Build history of the part. All positions in model axes, mm. A direction names the side the tool comes from. Round coordinates to 2 decimals unless told otherwise and drop trailing zeros. Write each loop counter-clockwise with the first axis right and the second up, starting at its lowest first coordinate (ties: lowest second). Pieces come first, ordered by that corner, then holes. Notation, with made-up numbers: (-35.5, 0.5) - (-10.5, 0.5) arc R18 cw to (-10.5, 17.5) - close; hole circle Ø2 at (55.5, 20). An arc over 180 degrees is marked (long way). Write each question's results on one line, items separated by ' | '.
from build123d import *

# Parameters (mm, degrees)
F0_W      = 90.9466184676
F0_H      = 74.8294964433
F2_DEPTH  = 5.08
F3_DEPTH  = 50.8
F5_DEPTH  = 76.2
F6_DEPTH  = 25.4
F8_DEPTH  = 101.6
F9_R      = 2.2127457179
F9_R_2    = 2.6181554233
F9_R_3    = 2.4324763665
F9_R_4    = 2.5640554726
F10_DEPTH = 25.4


with BuildPart() as f2:
    # F0 (on Front) → F2 (new body)
    with BuildSketch(Plane.XZ):
        with Locations((8.6341705173, 1.7268359661)):
            Rectangle(F0_W, F0_H)
    extrude(amount=F2_DEPTH)

    # F1 (on face) → F3 (join)
    with BuildSketch(Plane.XZ):
        Polygon((-27.9171578586, 32.2342440486), (-36.8391387165, 32.2342440486), (-36.8391387165, 2.734344452), (-36.5513302386, -26.7659369856), (-26.765935123, -26.7659369856), (-26.765935123, -34.8244979978), (43.1708656251, -34.8244979978), (43.1708656251, -26.4781285077), (54.1074797511, -26.4781285077), (54.1074797511, 31.0830231756), (42.5952523947, 31.0830231756), (42.5952523947, 39.1415841877), (-27.9171578586, 39.1415841877), align=None)
    extrude(amount=-F3_DEPTH)

    # F4 (on face) → F5 (cut)
    with BuildSketch(Plane.XY.offset(39.1415841877)):
        Polygon((-27.9171578586, 50.8), (-27.9171578586, 30.387243256), (12.6576088369, 14.234690927), (42.5952523947, 50.8), align=None)
    extrude(amount=-F5_DEPTH, mode=Mode.SUBTRACT)

    # F6 (cut): a face of the model
    f6_faces = [f2.faces().sort_by_distance(p)[0] for p in [
        (-32.3426594813, 50.8, 2.8940476275),
    ]]
    extrude(f6_faces, amount=-F6_DEPTH, mode=Mode.SUBTRACT)

    # F7 (on face) → F8 (cut)
    with BuildSketch(Plane(origin=(0, 0, -34.8244979978), x_dir=(1, 0, 0), z_dir=(0, 0, -1))):
        Polygon((-24.7789256071, -18.5888221988), (-22.6721912622, -24.9785389751), (9.4293939445, -12.1991054226), (6.9454660549, -5.9595469581), align=None)
    extrude(amount=-F8_DEPTH, mode=Mode.SUBTRACT)

    # F9 (on face) → F10 (cut)
    with BuildSketch(Plane(origin=(0, 0, 0), x_dir=(-1, 0, 0), z_dir=(0, 1, 0))):
        with Locations((32.3781482875, 36.15520522)):
            Circle(F9_R)
        with Locations((32.3781482875, -30.7667031884)):
            Circle(F9_R_2)
        with Locations((-49.00373891, -31.279515475)):
            Circle(F9_R_3)
        with Locations((-49.5165549219, 36.15520522)):
            Circle(F9_R_4)
    extrude(amount=-F10_DEPTH, mode=Mode.SUBTRACT)


solid = f2.part
(1) Slice it at A-A, the plane z = 18. Write the cut outline in (x, y), and give its area (3 significant figures).
Worked answers:
outline: (-36.84, -5.08) - (54.11, -5.08) - (54.11, 50.8) - (42.6, 50.8) - (12.66, 14.23) - (-27.92, 30.39) - (-27.92, 25.4) - (-36.84, 25.4) - close; hole (-24.78, 18.59) - (6.95, 5.96) - (9.43, 12.2) - (-22.67, 24.98) - close | area: 2,920 mm2
(2) Slice it at D-D, the plane x = -1.5. Write the cut outline in (y, z).
Worked answers:
outline: (-5.08, -35.69) - (0, -35.69) - (0, -34.82) - (9.32, -34.82) - (9.32, 39.14) - (-5.08, 39.14) - close; (16.55, -34.82) - (19.87, -34.82) - (19.87, 39.14) - (16.55, 39.14) - close
(3) Slice it at C-C, the plane y = 27.5. Write the cut outline in (x, z).
Worked answers:
outline: (-27.92, -26.77) - (-26.77, -26.77) - (-26.77, -34.82) - (-20.66, -34.82) - (-20.66, 39.14) - (-27.92, 39.14) - close; (23.52, -34.82) - (43.17, -34.82) - (43.17, -26.48) - (54.11, -26.48) - (54.11, 31.08) - (42.6, 31.08) - (42.6, 39.14) - (23.52, 39.14) - close
(4) Drill centre lines: probe 1 along Z at (x, y) = (33, 39); probe 2 along Y at (x, z) = (6, 21); probe 3 along Y at (x, z) = (-2.5, 12.5). Where is each one in solid material? Low to high. Write a range as [from, to].
Worked answers:
probe 1: z = [-34.82, 39.14] | probe 2: y = [-5.08, 6.34], [13.56, 16.89] | probe 3: y = [-5.08, 9.72], [16.95, 20.27]
(5) Two-plate mould, pull along Z, no slides. Class faces 1 (the flat face through (15, 14, -34.824)), 2 (the flat face through (54.107, 23, 1)), 3 (the flat face through (18, 11, 39.142)), 4 (the cylindrical face through (46.757, -2.504, -32.211)): released by +Z, released by -Z, zero draft, split by the parting line, or undercut.
Worked answers:
face 1: released by -Z | face 2: zero draft | face 3: released by +Z | face 4: undercut
(6) Tool access for faces 5 (the flat face through (48, 25, 31.083)), 6 (the flat face through (-7.914, 22.424, 2.676)), 7 (the flat face through (-32, 15, -26.766)), 8 (the flat face through (49, 25, -26.478)): list every direction of +Z, -Z, +X, -X, +Y, -Y with a clear straight run to the whole face (end or side of a thin tool).
Worked answers:
face 5: +Z, +X, +Y | face 6: +Z, -Z, +Y | face 7: -Z, -X, +Y | face 8: -Z, +X, +Y
(7) Flat gauge pins, fed straight in: pin 1 Ø2.5 at (x, z) = (47.5, 36.5) entering from +Y; pin 2 Ø4.5 at (x, z) = (-32.38, -30.77) entering from +Y; pin 3 Ø8 at (x, z) = (38.5, -5.5) entering from +Y; pin 4 Ø8.5 at (x, y) = (47.5, 19.5) entering from -Z. Where does each tip first touch, or does it go through?
Worked answers:
pin 1: stops at y = 0 | pin 2: passes through | pin 3: stops at y = 50.68 | pin 4: stops at z = -26.48
(8) Slice it at B-B, the plane x = 45.5. Write the cut outline in (y, z).
Worked answers:
outline: (-5.08, -35.69) - (0, -35.69) - (0, -26.48) - (50.8, -26.48) - (50.8, 31.08) - (0, 31.08) - (0, 39.14) - (-5.08, 39.14) - close
